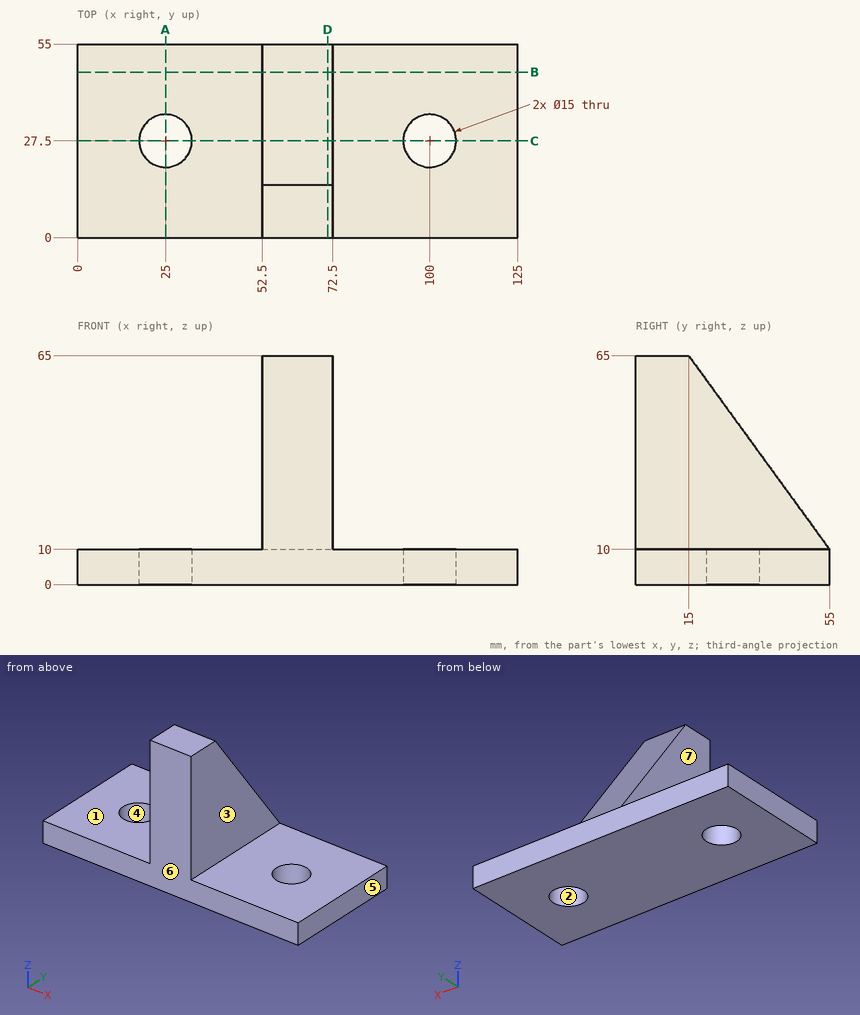
Geometry check sheet. Reference: drawing and pictorial views, mm from the part's lowest x, y, z. A direction names the side the tool comes from. Round coordinates to 2 decimals unless told otherwise and drop trailing zeros. Loops run counter-clockwise (first coordinate to the right, second up) from the corner with the lowest first, then second, coordinate; pieces in that order, holes last. Notation, with made-up numbers: (-12, -0.5) -> (44, -0.5) arc R25 cw to (44, 11.5) -> close; hole circle Ø6 at (21.5, 6). An arc over 180 degrees is marked (long way). Answer as a JSON object with one key per item and string values. Group by question number.
Item 1: Depth check by flat-ended pin: pin 1 Ø1.5 at (x, z) = (63.5, 19) entering from +Y; pin 2 Ø3 at (x, y) = (100.5, 32.5) entering from -Z; pin 3 Ø19.5 at (x, y) = (25, 27.5) entering from +Z. Enter the tip coordinate at first touch or a pass-through.
Item 2: Cross-section at C-C, the plane y = 27.5. Record the cut outline in (x, z), plus the area to 3 significant figures.
Item 3: Thickness scan on line 1 along X through (y, z) = (27, 7); line 2 along Y through (x, z) = (100, 4.75); line 3 along X through (y, z) = (30.5, 5.5). Record the ranges inside material, lowest first.
Item 4: Release check for a two-part mould opening along X. For the marked faces 4, 5, 6 and 7 record: pulls with the +X half, pulls with the -X half, needs draft (parallel to the pull), parting line crosses it, or undercut.
Item 5: Cross-section at D-D, the plane x = 71. Record the cut outline in (y, z).
Item 6: Cross-section at B-B, the plane y = 47. Record the cut outline in (x, z).
Item 7: Cross-section at A-A, the plane x = 25. Record the cut outline in (y, z).
Item 8: Set-up check for the marked faces 1, 2 and 3: record each of +Z, -Z, +X, -X, +Y, -Y from which the full face is reachable in a straight line by a thin tool's end or side.
Determined:
{
 "1": {"pin 1": "stops at y = 49", "pin 2": "passes through", "pin 3": "stops at z = 10"},
 "2": {"outline": "(0, 0) -> (17.5, 0) -> (17.5, 10) -> (0, 10) -> close; (32.5, 0) -> (92.5, 0) -> (92.5, 10) -> (72.5, 10) -> (72.5, 47.81) -> (52.5, 47.81) -> (52.5, 10) -> (32.5, 10) -> close; (107.5, 0) -> (125, 0) -> (125, 10) -> (107.5, 10) -> close", "area": "1,710 mm²"},
 "3": {"line 1": "x = 0 to 17.52, 32.48 to 92.52, 107.48 to 125", "line 2": "y = 0 to 20, 35 to 55", "line 3": "x = 0 to 18.13, 31.87 to 93.13, 106.87 to 125"},
 "4": {"face 4": "undercut", "face 5": "pulls with the +X half", "face 6": "needs draft", "face 7": "pulls with the -X half"},
 "5": {"outline": "(0, 0) -> (55, 0) -> (55, 10) -> (15, 65) -> (0, 65) -> close"},
 "6": {"outline": "(0, 0) -> (125, 0) -> (125, 10) -> (72.5, 10) -> (72.5, 21) -> (52.5, 21) -> (52.5, 10) -> (0, 10) -> close"},
 "7": {"outline": "(0, 0) -> (20, 0) -> (20, 10) -> (0, 10) -> close; (35, 0) -> (55, 0) -> (55, 10) -> (35, 10) -> close"},
 "8": {"face 1": "+Z, -X, +Y, -Y", "face 2": "+Z, -Z", "face 3": "+Z, +X, +Y, -Y"}
}
